Here's how the part is built. I have some questions about the finished solid (model axes, mm). A direction names the side the tool comes from. Round coordinates to 2 decimals unless told otherwise and drop trailing zeros. Loops run counter-clockwise (first coordinate to the right, second up) from the corner with the lowest first, then second, coordinate; pieces in that order, holes last. Notation, with made-up numbers: M 32,17.5 L 89,17.5 A20 ccw 89,43.5 Z; hole C -1.5,-23.5 d2. An arc over 180 degrees is marked long. Answer as a JSON object with one key per item and string values.
Autodesk Inventor part; units mm, degrees
ref_plane "Work Plane6" through (-134.9375, 20, -12.7) normal (0.3947, -0.9188, 0) x (0, 0, 1)
ref_plane "Work Plane7" through (-109.8713, -38.3432, -12.7) normal (0.3947, -0.9188, 0) x (0, 0, 1)
ref_plane "YZ Plane" through (0, 0, 0) normal (1, 0, 0) x (0, 1, 0)
sketch "Sketch1" plane through (0, 0, 0) normal (0, 1, 0) x (-1, 0, 0)
  circle A0 centre (0, 0) radius 135
  circle A1 centre (0, 0) radius 112.5
  dimension "d0" = 270
  dimension "d1" = 225
extrude "Extrusion1" add sketch "Sketch1" along normal mid plane 20
sketch "Sketch3" plane through (0, 10, 0) normal (0, 1, 0) x (1, 0, 0)
  circle A0 centre (0, 0) radius 125
  circle A1 centre (125, 0) radius 2.5
  circle A2 centre (101.1271, 73.4732) radius 2.5
  circle A3 centre (38.6271, 118.8821) radius 2.5
  circle A4 centre (-38.6271, 118.8821) radius 2.5
  circle A5 centre (-101.1271, 73.4732) radius 2.5
  circle A6 centre (-125, 0) radius 2.5
  circle A7 centre (-101.1271, -73.4732) radius 2.5
  circle A8 centre (-38.6271, -118.8821) radius 2.5
  circle A9 centre (38.6271, -118.8821) radius 2.5
  circle A10 centre (101.1271, -73.4732) radius 2.5
  dimension "d7" = 250
  dimension "d8" = 5
  dimension "d11" = 360
hole "Hole1" at (125, 10, 0) at (101.1271, 10, 73.4732) at (38.6271, 10, 118.8821) at (-38.6271, 10, 118.8821) at (-101.1271, 10, 73.4732) at (-125, 10, 0) at (-101.1271, 10, -73.4732) at (-38.6271, 10, -118.8821) at (38.6271, 10, -118.8821) at (101.1271, 10, -73.4732) direction (0, -1, 0) diameter 5 end through all
ref_plane "Work Plane6" through (-134.9375, 20, -12.7) normal (0.3947, -0.9188, 0) x (0, 0, 1)
ref_plane "Work Plane7" through (-109.8713, -38.3432, -12.7) normal (0.3947, -0.9188, 0) x (0, 0, 1)
sketch "Sketch5" plane through (-109.8713, -38.3432, -12.7) normal (0.3947, -0.9188, 0) x (0, 0, 1)
  circle A0 centre (12.7, -30.2265) radius 20
  point P0 (12.7, -116.0845)
  dimension "d26" = 40
  dimension "d27" = 85.858
extrude "Extrusion4" cut sketch "Sketch5" against normal blind 251.3
sketch "Sketch6" plane through (0, 0, 0) normal (1, 0, 0) x (0, 1, 0)
  line L0 (10, 15.5601) -> (10, -15.5601)
  line L1 (10, 0) -> (-10, 0)
  line L2 (-10, -2.5) -> (-10, 2.5)
  line L3 (11, -84.799) -> (1.1005, -74.8995)
  line L4 (11, -84.799) -> (25, -84.799) construction
  line L5 (11, -84.799) -> (11, -65)
  line L6 (1.1005, -74.8995) -> (1.1005, -65)
  line L7 (1.1005, -65) -> (11, -55.1005)
  line L8 (1.1005, -65) -> (15.1005, -65) construction
  line L9 (11, -55.1005) -> (11, -65)
  line L10 (11, 84.799) -> (1.1005, 74.8995)
  line L11 (11, 84.799) -> (25, 84.799) construction
  line L12 (11, 84.799) -> (11, 65)
  line L13 (1.1005, 74.8995) -> (1.1005, 65)
  line L14 (1.1005, 65) -> (11, 55.1005)
  line L15 (1.1005, 65) -> (15.1005, 65) construction
  line L16 (11, 55.1005) -> (11, 65)
  point P0 (0, 0)
  dimension "d30" = 14
  dimension "d31" = 135
  dimension "d34" = 65
  dimension "d35" = 14
  dimension "d36" = 45
extrude "Extrusion5" cut sketch "Sketch6" against normal through all
properties part number "Cylinder Spacer (x3)"
Item 1: I want a section at A-A, the plane z = -48. Please give me the cut outline in (x, y).
Resolved:
{"outline": "M -126.18,-10 L -101.75,-10 L -101.75,10 L -126.18,10 Z; M 101.75,-10 L 126.18,-10 L 126.18,10 L 101.75,10 Z"}
Item 2: I want a section at B-B, the plane x = 0. Please give me the cut outline in (y, z).
Resolved:
{"outline": "M -10,-135 L 10,-135 L 10,-112.5 L -10,-112.5 Z; M -10,112.5 L 10,112.5 L 10,135 L -10,135 Z"}
Item 3: I'm going to push flat-ended pins straight in: pin 1 Ø2 at (y, z) = (1, 106.5) entering from +X; pin 2 Ø8 at (x, z) = (-101.13, -73.47) entering from +Y; pin 3 Ø8 at (x, y) = (60.5, 6) entering from -Z. Where does each tip first touch, or does it pass through?
Resolved:
{"pin 1": "x = 84.23", "pin 2": "y = 3.67", "pin 3": "z = -122.61"}
Item 4: If we mould it in two halves opening along Z, with no side actions, what happens to faces 1 (the face through (112.39, -0.14, -4.95)), 2 (the face through (107.13, -0.14, 82.15)), 3 (the face through (113, 10, -9))? For each: pulls with the +Z half, pulls with the -Z half, needs draft (parallel to the pull), parting line crosses it, or undercut.
Resolved:
{"face 1": "undercut", "face 2": "parting line crosses it", "face 3": "needs draft"}
Item 5: On a 3-axis mill with a long thin cutter (end or side, diameter ignored), from which of +Z, -Z, +X, -X, +Y, -Y can I reach the whole of each face in a straight line? I mean faces 4 (the face through (-93.4, 5.6, -79.4)), 5 (the face through (-116.735, 3.547, 0.25)), 6 (the face through (-120, 10, 1)). Say none if no direction works.
Resolved:
{"face 4": "-X, +Y", "face 5": "+Y", "face 6": "+Z, -Z, +X, -X, +Y"}
Item 6: Please list where these lines run through material, in increasing order: probe 1 along X at (y, z) = (-5.75, -3); probe 2 along Z at (x, y) = (0, -3.75); probe 3 along X at (y, z) = (3, 26.5). Write a range as from..to.
Resolved:
{"probe 1": "-134.97..-112.5, 112.46..134.97", "probe 2": "-135..-112.5, 112.5..135", "probe 3": "-132.37..-109.33, 109.33..132.37"}
